For this review, take the finished solid that the model builds, in its own axes (mm). Face numbers are marked on the shaded views. Give positions to 0.01 mm unless a question says otherwise; leave off trailing zeros. Write each loop counter-clockwise with the first axis right and the second up, starting at its lowest first coordinate (ties: lowest second). Pieces come first, ordered by that corner, then holes. Notation, with made-up numbers: (-10, -7.5) -> (25, -7.5) arc R21 cw to (25, 6.5) -> close; hole circle Ø11 at (11.5, -34). An arc over 180 degrees is marked (long way). Write item = value, one per line.
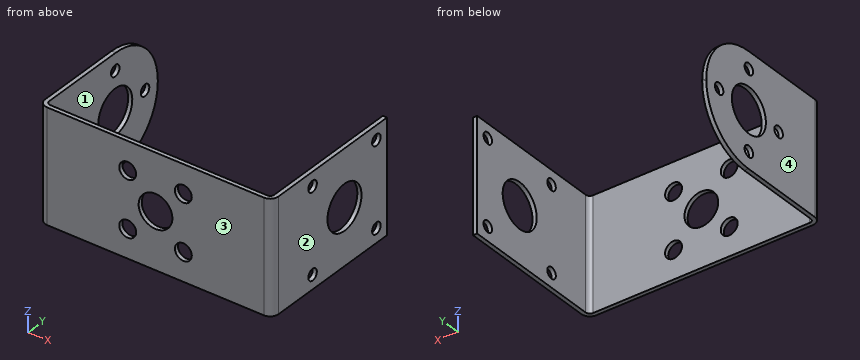
```python
from build123d import *

# Parameters (mm, degrees)
SKETCH_1_W                       = 41.5
SKETCH_1_H                       = 20
SKETCH_1_R                       = 3
SKETCH_1_R_2                     = 1.5
SM_BASE_FLANGE_1_DEPTH           = 0.7366
SM_EDGE_FLANGE_1_STRIP_W         = 4.4196
SM_EDGE_FLANGE_1_STRIP_H         = 0.7366
SM_EDGE_FLANGE_1_STRIP_CUT_DEPTH = 20
SM_EDGE_FLANGE_1_DEPTH           = 20
SM_EDGE_FLANGE_1_PROFILE_R       = 1
SM_EDGE_FLANGE_1_PROFILE_R_2     = 4
SM_EDGE_FLANGE_1_FLAT_DEPTH      = 0.7366
SM_EDGE_FLANGE_2_STRIP_W         = 4.4196
SM_EDGE_FLANGE_2_STRIP_H         = 0.7366
SM_EDGE_FLANGE_2_STRIP_CUT_DEPTH = 20
SM_EDGE_FLANGE_2_DEPTH           = 20
CUT_EXTRUDE_START                = -10
SKETCH_14_R                      = 4
SKETCH_14_R_2                    = 1
CUT_EXTRUDE_1_DEPTH              = 10


# Sheet-metal steps are written as plain solids
with BuildPart() as part:
    # Sketch 1 → 基体-法兰1 (new body)
    with BuildSketch(Plane(origin=(0, 0, 0), x_dir=(1, 0, 0), z_dir=(0, 1, 0))):
        Rectangle(SKETCH_1_W, SKETCH_1_H)
        with Locations(Location((0, 0, 0), (0, 0, 270))):
            Circle(SKETCH_1_R, mode=Mode.SUBTRACT)
        with Locations(Location((4.9495, 4.9495, 0), (0, 0, 270))):
            Circle(SKETCH_1_R_2, mode=Mode.SUBTRACT)
        with Locations(Location((-4.9495, 4.9495, 0), (0, 0, 270))):
            Circle(SKETCH_1_R_2, mode=Mode.SUBTRACT)
        with Locations(Location((-4.9495, -4.9495, 0), (0, 0, 270))):
            Circle(SKETCH_1_R_2, mode=Mode.SUBTRACT)
        with Locations(Location((4.9495, -4.9495, 0), (0, 0, 270))):
            Circle(SKETCH_1_R_2, mode=Mode.SUBTRACT)
    extrude(amount=-SM_BASE_FLANGE_1_DEPTH)

    # 边线-法兰1 strip (across the edge) → 边线-法兰1 strip cut (cut)
    with BuildSketch(Plane(origin=(-20.75, 0, -10), x_dir=(1, 0, 0), z_dir=(0, 0, 1))):
        with Locations((-0.7366, -0.3683)):
            Rectangle(SM_EDGE_FLANGE_1_STRIP_W, SM_EDGE_FLANGE_1_STRIP_H)
    extrude(amount=SM_EDGE_FLANGE_1_STRIP_CUT_DEPTH, mode=Mode.SUBTRACT)

    # 边线-法兰1 bend section (across the edge) → 边线-法兰1 (add)
    with BuildSketch(Plane(origin=(-20.75, 0, -10), x_dir=(1, 0, 0), z_dir=(0, 0, 1))):
        with BuildLine():
            Line((0, 0.7366), (0.7366, 0.7366))
            ThreePointArc((0.7366, 0.7366), (0.952345145, 0.215745145), (1.4732, 0))
            Line((1.4732, 0), (1.4732, -0.7366))
            ThreePointArc((1.4732, -0.7366), (0.43149029, -0.30510971), (0, 0.7366))
        make_face()
    extrude(amount=SM_EDGE_FLANGE_1_DEPTH)

    # 边线-法兰1 profile (on flange) → 边线-法兰1 flat (add)
    with BuildSketch(Plane.ZY.offset(20.75)):
        with BuildLine():
            Line((-10, 0.7366), (10, 0.7366))
            Line((10, 0.7366), (10, 16.3634))
            ThreePointArc((10, 16.3634), (7.100357134, 23.363757134), (0.1, 26.2634))
            Line((0.1, 26.2634), (-0.1, 26.2634))
            ThreePointArc((-0.1, 26.2634), (-7.100357134, 23.363757134), (-10, 16.3634))
            Line((-10, 16.3634), (-10, 0.7366))
        make_face()
        with Locations((0, 9.2634)):
            Circle(SM_EDGE_FLANGE_1_PROFILE_R, mode=Mode.SUBTRACT)
        with Locations((7, 16.2634)):
            Circle(SM_EDGE_FLANGE_1_PROFILE_R, mode=Mode.SUBTRACT)
        with Locations((0, 16.2634)):
            Circle(SM_EDGE_FLANGE_1_PROFILE_R_2, mode=Mode.SUBTRACT)
        with Locations((-7, 16.2634)):
            Circle(SM_EDGE_FLANGE_1_PROFILE_R, mode=Mode.SUBTRACT)
        with Locations((0, 23.2634)):
            Circle(SM_EDGE_FLANGE_1_PROFILE_R, mode=Mode.SUBTRACT)
    extrude(amount=-SM_EDGE_FLANGE_1_FLAT_DEPTH)

    # 边线-法兰2 strip (across the edge) → 边线-法兰2 strip cut (cut)
    with BuildSketch(Plane(origin=(20.75, 0, 10), x_dir=(-1, 0, 0), z_dir=(0, 0, -1))):
        with Locations((-0.7366, -0.3683)):
            Rectangle(SM_EDGE_FLANGE_2_STRIP_W, SM_EDGE_FLANGE_2_STRIP_H)
    extrude(amount=SM_EDGE_FLANGE_2_STRIP_CUT_DEPTH, mode=Mode.SUBTRACT)

    # 边线-法兰2 section (across the edge) → 边线-法兰2 (add)
    with BuildSketch(Plane(origin=(20.75, 0, 10), x_dir=(-1, 0, 0), z_dir=(0, 0, -1))):
        with BuildLine():
            Line((0, 0.7366), (0, 26.2634))
            Line((0, 26.2634), (0.7366, 26.2634))
            Line((0.7366, 26.2634), (0.7366, 0.7366))
            ThreePointArc((0.7366, 0.7366), (0.952345145, 0.215745145), (1.4732, 0))
            Line((1.4732, 0), (1.4732, -0.7366))
            ThreePointArc((1.4732, -0.7366), (0.43149029, -0.30510971), (0, 0.7366))
        make_face()
    extrude(amount=SM_EDGE_FLANGE_2_DEPTH)

    # 草图14 → 切除-拉伸1 (cut)
    with BuildSketch(Plane(origin=(20.75, 0, 0), x_dir=(0, 0, -1), z_dir=(1, 0, 0)).offset(CUT_EXTRUDE_START)):
        with Locations(Location((0, 16.2634, 0), (0, 0, 90))):
            Circle(SKETCH_14_R)
        with Locations(Location((-7.5, 23.7634, 0), (0, 0, 90))):
            Circle(SKETCH_14_R_2)
        with Locations(Location((7.5, 23.7634, 0), (0, 0, 90))):
            Circle(SKETCH_14_R_2)
        with Locations(Location((7.5, 8.7634, 0), (0, 0, 90))):
            Circle(SKETCH_14_R_2)
        with Locations(Location((-7.5, 8.7634, 0), (0, 0, 90))):
            Circle(SKETCH_14_R_2)
    extrude(amount=CUT_EXTRUDE_1_DEPTH, mode=Mode.SUBTRACT)


solid = part.part
```
(1) Take a section at B-B (z = -7). Write out the cut boundary in (x, y).
Answers below:
outline = (-20.75, 0.74) arc R1.47 ccw to (-19.28, -0.74) -> (19.28, -0.74) arc R1.47 ccw to (20.75, 0.74) -> (20.75, 7.9) -> (20.01, 7.9) -> (20.01, 0.74) arc R0.74 cw to (19.28, 0) -> (-19.28, 0) arc R0.74 cw to (-20.01, 0.74) -> (-20.01, 15.26) -> (-20.75, 15.26) -> close; (-20.75, 17.26) -> (-20.01, 17.26) -> (-20.01, 23.46) -> (-20.75, 23.46) -> close; (20.01, 9.63) -> (20.75, 9.63) -> (20.75, 22.9) -> (20.01, 22.9) -> close; (20.01, 24.63) -> (20.75, 24.63) -> (20.75, 26.26) -> (20.01, 26.26) -> close
(2) Take a section at D-D (y = 14.5). Write out the cut boundary in (x, z), plus the area to 3 significant figures.
Answers below:
outline = (-20.75, -10) -> (-20.01, -10) -> (-20.01, -3.59) -> (-20.75, -3.59) -> close; (-20.75, 3.59) -> (-20.01, 3.59) -> (-20.01, 10) -> (-20.75, 10) -> close; (20.01, -10) -> (20.75, -10) -> (20.75, -3.59) -> (20.01, -3.59) -> close; (20.01, 3.59) -> (20.75, 3.59) -> (20.75, 10) -> (20.01, 10) -> close
area = 18.9 mm^2
(3) For pin 1 (3 mm diameter, centred on x = 12, z = 3, fed in from +Y); pin 2 (7 mm diameter, centred on x = 0, z = 0, fed in from -Y); pin 3 (1.2 mm diameter, centred on y = 23.76, z = -7.5, fed in from +X), all flat-tipped, find the tip position at first contact; note any pin that passes through.
Answers below:
pin_1 = 0
pin_2 = -0.74
pin_3 = -20.01
(4) Take a section at C-C (y = 21.5). Write out the cut boundary in (x, z), plus the area to 3 significant figures.
Answers below:
outline = (-20.75, -8.56) -> (-20.01, -8.56) -> (-20.01, 8.56) -> (-20.75, 8.56) -> close; (20.01, -10) -> (20.75, -10) -> (20.75, 10) -> (20.01, 10) -> close
area = 27.3 mm^2
(5) The part is to be moulded in two halves that separate along X. For the marked faces 1, 2, 3 and 4, say which applies: released by +X, released by -X, zero draft, split by the parting line, or undercut.
Answers below:
face_1 = undercut
face_2 = released by +X
face_3 = zero draft
face_4 = released by -X
(6) Take a section at A-A (x = 0). Write out the cut boundary in (y, z).
Answers below:
outline = (-0.74, -10) -> (0, -10) -> (0, -3) -> (-0.74, -3) -> close; (-0.74, 3) -> (0, 3) -> (0, 10) -> (-0.74, 10) -> close
(7) To check wall thickness, follow probe 1 along X at (y, z) = (9.75, -4.5); probe 2 along Y at (x, z) = (-20.5, 0); probe 3 along Y at (x, z) = (8, 8). State the ranges of each line that lie inside material, in increasing order.
Answers below:
probe_1 = -20.75 to -20.01, 20.01 to 20.75
probe_2 = -0.08 to 8.26, 10.26 to 12.26, 20.26 to 22.26, 24.26 to 26.26
probe_3 = -0.74 to 0
